from build123d import *

# Parameters (mm, degrees)
SKETCH1_W                = 50
SKETCH1_H                = 25
BOSS_EXTRUDE1_DEPTH      = 25
BOSS_EXTRUDE2_DEPTH      = 25
SKETCH4_R                = 6.625
CUT_EXTRUDE1_DEPTH       = 75
SKETCH9_R                = 3.1
CUT_EXTRUDE6_DEPTH       = 116.938210964
FILLET3_R                = 5
FILLET5_R                = 3
SKETCH10_W               = 47.732743957
SKETCH10_H               = 107.667843513
CUT_EXTRUDE7_DEPTH       = 100
SKETCH11_W               = 28.236029243
SKETCH11_H               = 25
CUT_EXTRUDE8_DEPTH       = 111.285013225
SKETCH12_W               = 27.477268163
SKETCH12_H               = 27.699456316
CUT_EXTRUDE9_DEPTH       = 5
BODY_MOVE_COPY1_ANGLE    = 8
SKETCH13_W               = 22.608001889
SKETCH13_H               = 25
BOSS_EXTRUDE3_DEPTH      = 29
SKETCH14_W               = 25
SKETCH14_H               = 20
BOSS_EXTRUDE4_DEPTH      = 74.967411564
CUT_EXTRUDE10_DEPTH      = 113.041997451
CUT_EXTRUDE10_DEPTH_BACK = 113.041997451
SKETCH15_R               = 4.7625
SKETCH15_R_2             = 3.1


with BuildPart() as part:
    # Sketch1 → Boss-Extrude1 (new body)
    with BuildSketch(Plane.XY):
        Rectangle(SKETCH1_W, SKETCH1_H)
    extrude(amount=BOSS_EXTRUDE1_DEPTH)

    # Sketch3 → Boss-Extrude2 (add)
    with BuildSketch(Plane.XY.offset(25)):
        Polygon((-25, 12.5), (-99.270105156, 22.937982572), (-95.929950733, 46.704416222), (-25, 36.73586174), (-25, 31.73586174), (25, 31.73586174), (25, 36.73586174), (95.929950733, 46.704416222), (99.270105156, 22.937982572), (25, 12.5), align=None)
    extrude(amount=-BOSS_EXTRUDE2_DEPTH)

    # Sketch4 → Cut-Extrude1 (cut)
    with BuildSketch(Plane(origin=(-100.508609829, 14.12556392, 0), x_dir=(0, 0, 1), z_dir=(-0.9902680687415705, 0.13917310096006502, 0))):
        with Locations(Location((12.5, 20.899023335, 0), (0, 0, 270))):
            Circle(SKETCH4_R)
    cut_extrude1 = extrude(amount=-CUT_EXTRUDE1_DEPTH, mode=Mode.SUBTRACT)

    # Mirror1: Cut-Extrude1 across plane
    add(cut_extrude1.mirror(Plane(origin=(0, 0, 0), x_dir=(0, 0, 1), z_dir=(1, 0, 0))), mode=Mode.SUBTRACT)

    # Sketch9 → Cut-Extrude6 (cut, through all)
    with BuildSketch(Plane(origin=(4.578659096, 32.578852302, 0), x_dir=(0.9902680687415703, -0.1391731009600656, 0), z_dir=(0.1391731009600656, 0.9902680687415703, 0))):
        with Locations(Location((-91.496365481, -12.5, 0), (0, 0, 180))):
            Circle(SKETCH9_R)
        with Locations(Location((-71.496365481, -12.5, 0), (0, 0, 180))):
            Circle(SKETCH9_R)
        with Locations(Location((-51.496365481, -12.5, 0), (0, 0, 180))):
            Circle(SKETCH9_R)
    extrude(amount=-CUT_EXTRUDE6_DEPTH, mode=Mode.SUBTRACT)

    # Fillet3
    # the kernel refuses this fillet: 5 mm, written as the material it takes off along each edge
    with BuildSketch(Plane(origin=(111.648456015, 24.677646334, 25), x_dir=(-0.13917310096006577, 0.9902680687415704, 0), z_dir=(-0.9902680687415703, -0.13917310096006574, 0))) as fillet3_piece_1_section:
        with BuildLine():
            CenterArc((FILLET3_R, FILLET3_R), FILLET3_R, 180, 90)
            Line((0, FILLET3_R), (0, 0))
            Line((0, 0), (FILLET3_R, 0))
        make_face()
    fillet3_piece_1 = extrude(amount=100, mode=Mode.PRIVATE)
    fillet3_piece_1 = split(fillet3_piece_1, bisect_by=Plane(origin=(25, 18.834233779, 23.882189323), z_dir=(1, 0, 0)), keep=Keep.TOP, mode=Mode.PRIVATE)
    add(fillet3_piece_1, mode=Mode.SUBTRACT)
    with BuildSketch(Plane(origin=(12.621649141, 34.996197978, 25), x_dir=(0.13917310096006597, -0.9902680687415704, 0), z_dir=(0.9902680687415703, 0.13917310096006597, 0))) as fillet3_piece_2_section:
        with BuildLine():
            CenterArc((FILLET3_R, FILLET3_R), FILLET3_R, 180, 90)
            Line((0, FILLET3_R), (0, 0))
            Line((0, 0), (FILLET3_R, 0))
        make_face()
    fillet3_piece_2 = extrude(amount=96.627019967, mode=Mode.PRIVATE)
    fillet3_piece_2 = split(fillet3_piece_2, bisect_by=Plane(origin=(60.542812169, 31.73586174, 23.884172665), z_dir=(0, 1, 0)), keep=Keep.TOP, mode=Mode.PRIVATE)
    add(fillet3_piece_2, mode=Mode.SUBTRACT)
    with BuildSketch(Plane(origin=(-108.308301592, 48.444079984, 25), x_dir=(-0.13917310096006566, -0.9902680687415704, 0), z_dir=(0.9902680687415704, -0.13917310096006566, 0))) as fillet3_piece_3_section:
        with BuildLine():
            CenterArc((FILLET3_R, FILLET3_R), FILLET3_R, 180, 90)
            Line((0, FILLET3_R), (0, 0))
            Line((0, 0), (FILLET3_R, 0))
        make_face()
    fillet3_piece_3 = extrude(amount=96.627019967, mode=Mode.PRIVATE)
    fillet3_piece_3 = split(fillet3_piece_3, bisect_by=Plane(origin=(-60.542812169, 31.73586174, 23.884172665), z_dir=(0, 1, 0)), keep=Keep.TOP, mode=Mode.PRIVATE)
    add(fillet3_piece_3, mode=Mode.SUBTRACT)
    with BuildSketch(Plane(origin=(-12.621649141, 10.760336238, 25), x_dir=(0.13917310096006563, 0.9902680687415704, 0), z_dir=(-0.9902680687415703, 0.13917310096006563, 0))) as fillet3_piece_4_section:
        with BuildLine():
            CenterArc((FILLET3_R, FILLET3_R), FILLET3_R, 180, 90)
            Line((0, FILLET3_R), (0, 0))
            Line((0, 0), (FILLET3_R, 0))
        make_face()
    fillet3_piece_4 = extrude(amount=100, mode=Mode.PRIVATE)
    fillet3_piece_4 = split(fillet3_piece_4, bisect_by=Plane(origin=(-25, 18.834233779, 23.882189323), z_dir=(-1, 0, 0)), keep=Keep.TOP, mode=Mode.PRIVATE)
    add(fillet3_piece_4, mode=Mode.SUBTRACT)
    with BuildSketch(Plane(origin=(111.648456015, 24.677646334, 0), x_dir=(-0.13917310096006577, 0.9902680687415704, 0), z_dir=(-0.9902680687415703, -0.13917310096006574, 0))) as fillet3_piece_5_section:
        with BuildLine():
            CenterArc((FILLET3_R, -FILLET3_R), FILLET3_R, 90, 90)
            Line((0, -FILLET3_R), (0, 0))
            Line((0, 0), (FILLET3_R, 0))
        make_face()
    fillet3_piece_5 = extrude(amount=100, mode=Mode.PRIVATE)
    fillet3_piece_5 = split(fillet3_piece_5, bisect_by=Plane(origin=(25, 18.834233779, 1.117810677), z_dir=(1, 0, 0)), keep=Keep.TOP, mode=Mode.PRIVATE)
    add(fillet3_piece_5, mode=Mode.SUBTRACT)
    with BuildSketch(Plane(origin=(12.621649141, 34.996197978, 0), x_dir=(0.13917310096006597, -0.9902680687415704, 0), z_dir=(0.9902680687415703, 0.13917310096006597, 0))) as fillet3_piece_6_section:
        with BuildLine():
            CenterArc((FILLET3_R, -FILLET3_R), FILLET3_R, 90, 90)
            Line((0, -FILLET3_R), (0, 0))
            Line((0, 0), (FILLET3_R, 0))
        make_face()
    fillet3_piece_6 = extrude(amount=96.627019967, mode=Mode.PRIVATE)
    fillet3_piece_6 = split(fillet3_piece_6, bisect_by=Plane(origin=(60.542812169, 31.73586174, 1.115827335), z_dir=(0, 1, 0)), keep=Keep.TOP, mode=Mode.PRIVATE)
    add(fillet3_piece_6, mode=Mode.SUBTRACT)
    with BuildSketch(Plane(origin=(-108.308301592, 48.444079984, 0), x_dir=(-0.13917310096006566, -0.9902680687415704, 0), z_dir=(0.9902680687415704, -0.13917310096006566, 0))) as fillet3_piece_7_section:
        with BuildLine():
            CenterArc((FILLET3_R, -FILLET3_R), FILLET3_R, 90, 90)
            Line((0, -FILLET3_R), (0, 0))
            Line((0, 0), (FILLET3_R, 0))
        make_face()
    fillet3_piece_7 = extrude(amount=96.627019967, mode=Mode.PRIVATE)
    fillet3_piece_7 = split(fillet3_piece_7, bisect_by=Plane(origin=(-60.542812169, 31.73586174, 1.115827335), z_dir=(0, 1, 0)), keep=Keep.TOP, mode=Mode.PRIVATE)
    add(fillet3_piece_7, mode=Mode.SUBTRACT)
    with BuildSketch(Plane(origin=(-12.621649141, 10.760336238, 0), x_dir=(0.13917310096006563, 0.9902680687415704, 0), z_dir=(-0.9902680687415703, 0.13917310096006563, 0))) as fillet3_piece_8_section:
        with BuildLine():
            CenterArc((FILLET3_R, -FILLET3_R), FILLET3_R, 90, 90)
            Line((0, -FILLET3_R), (0, 0))
            Line((0, 0), (FILLET3_R, 0))
        make_face()
    fillet3_piece_8 = extrude(amount=100, mode=Mode.PRIVATE)
    fillet3_piece_8 = split(fillet3_piece_8, bisect_by=Plane(origin=(-25, 18.834233779, 1.117810677), z_dir=(-1, 0, 0)), keep=Keep.TOP, mode=Mode.PRIVATE)
    add(fillet3_piece_8, mode=Mode.SUBTRACT)

    # Fillet5
    fillet5_edges = [part.edges().sort_by_distance(p)[0] for p in [
        (25, 31.73586174, 12.5),
        (-25, 31.73586174, 12.5),
    ]]
    fillet(fillet5_edges, radius=FILLET5_R)

    # Sketch10 → Cut-Extrude7 (cut)
    with BuildSketch(Plane(origin=(0, 0, 0), x_dir=(0, 0, -1), z_dir=(1, 0, 0))):
        with Locations((-11.782214376, 4.002620484)):
            Rectangle(SKETCH10_W, SKETCH10_H)
    extrude(amount=CUT_EXTRUDE7_DEPTH, mode=Mode.SUBTRACT)

    # Sketch11 → Cut-Extrude8 (cut, through all)
    with BuildSketch(Plane(origin=(1.238504673, 8.812418652, 0), x_dir=(0.9902680687415703, -0.13917310096006563, 0), z_dir=(-0.13917310096006563, -0.9902680687415703, 0))):
        with Locations((-12.37835086, 12.5)):
            Rectangle(SKETCH11_W, SKETCH11_H)
    extrude(amount=CUT_EXTRUDE8_DEPTH, mode=Mode.SUBTRACT)

    # Sketch12 → Cut-Extrude9 (cut)
    with BuildSketch(Plane(origin=(4.578659096, 32.578852302, 0), x_dir=(0.9902680687415703, -0.1391731009600656, 0), z_dir=(0.1391731009600656, 0.9902680687415703, 0))):
        with Locations((-12.790319835, -12.604422979)):
            Rectangle(SKETCH12_W, SKETCH12_H)
    extrude(amount=-CUT_EXTRUDE9_DEPTH, mode=Mode.SUBTRACT)


with BuildPart() as part_1:
    # Body-Move/Copy1: moved
    add(part.part.rotate(Axis((-49.635052578, 27.845447677, 0), (0, 0, 1)), BODY_MOVE_COPY1_ANGLE))

    # Sketch13 → Boss-Extrude3 (add)
    with BuildSketch(Plane(origin=(0, 35.077877501, 0), x_dir=(1, 0, 0), z_dir=(0, 1, 0))):
        with Locations((-11.832660591, -12.5)):
            Rectangle(SKETCH13_W, SKETCH13_H)
    extrude(amount=BOSS_EXTRUDE3_DEPTH)

    # Sketch14 → Boss-Extrude4 (add)
    with BuildSketch(Plane.ZY.offset(23.136661535)):
        with Locations((12.5, 54.077877501)):
            Rectangle(SKETCH14_W, SKETCH14_H)
    extrude(amount=BOSS_EXTRUDE4_DEPTH)

    # Sketch15 → Cut-Extrude10 (cut, two sides: drawn at the far end of the back side and taken through both)
    # profile 1 of 6: a face of its own
    with BuildSketch(Plane(origin=(0, 64.077877501, 0), x_dir=(1, 0, 0), z_dir=(0, 1, 0)).offset(-CUT_EXTRUDE10_DEPTH_BACK)):
        with Locations(Location((-88.104073099, -12.5, 0), (0, 0, 270))):
            Circle(SKETCH15_R)
        with Locations((-88.104073099, -12.5)):
            Circle(SKETCH15_R_2, mode=Mode.SUBTRACT)
    # profile 2 of 6: a face of its own
    with BuildSketch(Plane(origin=(0, 64.077877501, 0), x_dir=(1, 0, 0), z_dir=(0, 1, 0)).offset(-CUT_EXTRUDE10_DEPTH_BACK)):
        with Locations((-88.104073099, -12.5)):
            Circle(SKETCH15_R_2)
    # profile 3 of 6: a face of its own
    with BuildSketch(Plane(origin=(0, 64.077877501, 0), x_dir=(1, 0, 0), z_dir=(0, 1, 0)).offset(-CUT_EXTRUDE10_DEPTH_BACK)):
        with Locations(Location((-68.104073099, -12.5, 0), (0, 0, 270))):
            Circle(SKETCH15_R)
        with Locations((-68.104073099, -12.5)):
            Circle(SKETCH15_R_2, mode=Mode.SUBTRACT)
    # profile 4 of 6: a face of its own
    with BuildSketch(Plane(origin=(0, 64.077877501, 0), x_dir=(1, 0, 0), z_dir=(0, 1, 0)).offset(-CUT_EXTRUDE10_DEPTH_BACK)):
        with Locations((-68.104073099, -12.5)):
            Circle(SKETCH15_R_2)
    # profile 5 of 6: a face of its own
    with BuildSketch(Plane(origin=(0, 64.077877501, 0), x_dir=(1, 0, 0), z_dir=(0, 1, 0)).offset(-CUT_EXTRUDE10_DEPTH_BACK)):
        with Locations(Location((-48.104073099, -12.5, 0), (0, 0, 270))):
            Circle(SKETCH15_R)
        with Locations((-48.104073099, -12.5)):
            Circle(SKETCH15_R_2, mode=Mode.SUBTRACT)
    # profile 6 of 6: a face of its own
    with BuildSketch(Plane(origin=(0, 64.077877501, 0), x_dir=(1, 0, 0), z_dir=(0, 1, 0)).offset(-CUT_EXTRUDE10_DEPTH_BACK)):
        with Locations((-48.104073099, -12.5)):
            Circle(SKETCH15_R_2)
    extrude(amount=CUT_EXTRUDE10_DEPTH + CUT_EXTRUDE10_DEPTH_BACK, mode=Mode.SUBTRACT)


solid = part_1.part
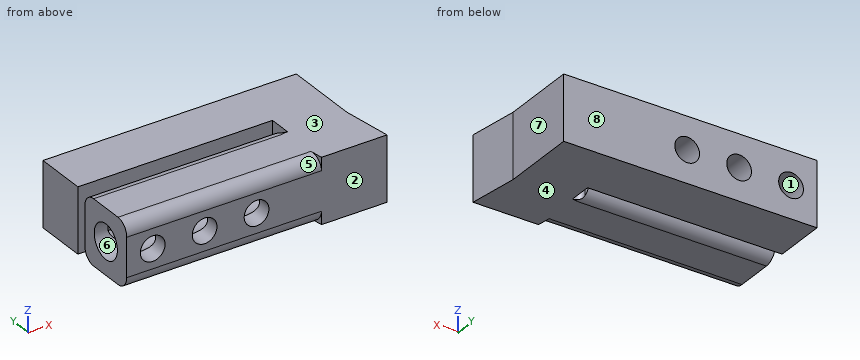
Part model, mm, in its own coordinate system. Face numbers are marked on the shaded views. A direction names the side the tool comes from. Coordinates: 2 decimals unless noted, no trailing zeros. Loops run counter-clockwise (first coordinate to the right, second up) from the corner with the lowest first, then second, coordinate; pieces in that order, holes last. Notation, with made-up numbers: (81, 57) -> (85, 57) arc R31 ccw to (85, 95) -> close; hole circle Ø11 at (55.5, 61). An arc over 180 degrees is marked (long way). Use a Markdown table: item, result. Add a question column.
Item 1: Band-saw the part on B-B on y = 55. Write the cut outline in (x, z) (1 decimal).
Item 2: Which spindle directions (+Z, -Z, +X, -X, +Y, -Y) get a long thin tool onto all of the face, cutting with end or side? Do the marked faces 5, 6, 7 and 8. Say none if no direction does.
Item 3: Flat gauge pins, fed straight in: P1, Ø11, axis at x = -48.1, z = 12.5, coming from the -Y side; P2, Ø12.5, axis at y = 56.5, z = 15.5, coming from the +X side; P3, Ø10.5, axis at y = 28.08, z = 12.5, coming from the +X side; P4, Ø1, axis at y = 22, z = 10, coming from the +X side. Where does each tip first touch, or does it go through?
Item 4: Band-saw the part on C-C on x = -66. Give the number of separate pieces and of enclosed holes in the cut face, plus the area to 3 significant figures.
Item 5: Pull direction Z, two halves, no side cores. Call the marked faces 1, 2, 3 and 4: +Z half, -Z half, draft (parallel to the pull), parting line (faces both ways), or undercut.
Item 6: Band-saw the part on A-A on x = -40.5. Write the cut outline in (y, z) (3 decimals), plus the area to 3 significant figures.
Item 7: Probe probe 1 along Y at (x, z) = (-41.5, 12); probe 2 along Y at (x, z) = (-36.5, 7.75); probe 3 along X at (y, z) = (35.75, 12.5). List the from-to ranges inside material, lowest first.
Geometry says:
| question | item | result |
|---|---|---|
| 1 | outline | (-98.1, 0) -> (-0.5, 0) -> (-0.5, 25) -> (-98.1, 25) -> close; hole circle Ø9.5 at (-88.1, 12.5); hole circle Ø9.5 at (-68.1, 12.5); hole circle Ø9.5 at (-48.1, 12.5) |
| 2 | face 5 | +Z, -X, -Y |
| 2 | face 6 | -X |
| 2 | face 7 | +Z, -Z, +X, +Y |
| 2 | face 8 | +Z, -Z, +X, -X, +Y |
| 3 | P1 | y = 16.08 |
| 3 | P2 | x = -0.53 |
| 3 | P3 | x = 1.19 |
| 3 | P4 | x = 1.38 |
| 4 | separate pieces | 4 |
| 4 | enclosed holes | 0 |
| 4 | area | 669 mm² |
| 5 | face 1 | undercut |
| 5 | face 2 | draft |
| 5 | face 3 | +Z half |
| 5 | face 4 | -Z half |
| 6 | outline | (16.078, 5) arc R5 ccw to (21.078, 0) -> (35.078, 0) arc R5 ccw to (40.078, 5) -> (40.078, 20) arc R5 ccw to (35.078, 25) -> (21.078, 25) arc R5 ccw to (16.078, 20) -> close; (44.078, 0) -> (64.078, 0) -> (64.078, 25) -> (44.078, 25) -> close; hole circle Ø13.25 at (28.078, 12.5) |
| 6 | area | 941 mm² |
| 7 | probe 1 | 16.08 to 21.47, 34.68 to 40.08, 44.08 to 64.08 |
| 7 | probe 2 | 16.08 to 23.46, 32.7 to 40.08, 44.08 to 64.08 |
| 7 | probe 3 | -98.1 to -92.87, -83.34 to -72.87, -63.34 to -52.87, -43.34 to -24.39, -23.14 to -0.53 |
